Source: CAD feature listing. Evaluate the final solid. Frame: model axes, mm. A direction names the side the tool comes from. Give positions to 0.01 mm unless a question says otherwise; leave off trailing zeros. Order: outer loops, then holes, each group sorted by start corner. A loop starts at its lowest first (then second) coordinate and runs counter-clockwise, first axis right, second up. Notation, with made-up numbers: (54.25, -40) -> (69.25, -40) arc R20 cw to (69.25, -33) -> close; hole circle Ø10 at (84.5, -5.5). An arc over 180 degrees is marked (long way). Use CSV: the item, a comma, the result in double quotes.
```python
from build123d import *

# Parameters (mm, degrees)
SKETCH_1_R          = 2.1
EXTRUDE_1_DEPTH     = 5
SKETCH_2_R          = 3.75
EXTRUDE_2_DEPTH     = 4.2
SKETCH_3_R          = 4.35
EXTRUDE_3_DEPTH     = 1
SKETCH_9_R          = 2.5
CUT_EXTRUDE_1_DEPTH = 2.5


with BuildPart() as part:
    # 스케치1 → 보스-돌출1 (new body)
    with BuildSketch(Plane.XY):
        Circle(SKETCH_1_R)
    extrude(amount=EXTRUDE_1_DEPTH)

    # 스케치2 → 보스-돌출2 (add)
    with BuildSketch(Plane.XY.offset(5)):
        Circle(SKETCH_2_R)
    extrude(amount=EXTRUDE_2_DEPTH)

    # 스케치3 → 보스-돌출3 (add)
    with BuildSketch(Plane.XY.offset(9.2)):
        Circle(SKETCH_3_R)
    extrude(amount=EXTRUDE_3_DEPTH)

    # 스케치9 → 컷-돌출1 (cut)
    with BuildSketch(Plane.XY.offset(10.2)):
        Circle(SKETCH_9_R)
    extrude(amount=-CUT_EXTRUDE_1_DEPTH, mode=Mode.SUBTRACT)

    # 스케치13 → M2 남비 머리 나사용 카운터보어2 (revolve, cut)
    with BuildSketch(Plane(origin=(0, 0, 7.7), x_dir=(0, -1, 0), z_dir=(1, 0, 0))):
        Polygon((0, 0), (0, 8.781118805), (1.3, 8), (1.3, 1.6), (2.5, 1.6), (2.5, 0.025), (2.525, 0), align=None)
    revolve(axis=Axis((0, 0, 14.05), (0, 0, -1)), mode=Mode.SUBTRACT)


solid = part.part
```
1. Section query A-A on y = 0. Return loops of the section in (x, z) (3 decimals), plus the area to 3 significant figures.
Answer below:
outline,"(-4.35, 9.2) -> (-3.75, 9.2) -> (-3.75, 5) -> (-2.1, 5) -> (-2.1, 0) -> (-1.3, 0) -> (-1.3, 6.1) -> (-2.5, 6.1) -> (-2.5, 7.675) -> (-2.525, 7.7) -> (-2.5, 7.7) -> (-2.5, 10.2) -> (-4.35, 10.2) -> close; (1.3, 0) -> (2.1, 0) -> (2.1, 5) -> (3.75, 5) -> (3.75, 9.2) -> (4.35, 9.2) -> (4.35, 10.2) -> (2.5, 10.2) -> (2.5, 7.7) -> (2.525, 7.7) -> (2.5, 7.675) -> (2.5, 6.1) -> (1.3, 6.1) -> close"
area,"24.8 mm²"
2. Ray query, line 1 along Y through (x, z) = (0, 3.25); line 2 along Y through (x, z) = (0, 8.75); line 3 along Z through (x, y) = (-2.75, -0.75). Return the intervals inside material, ascending.
Answer below:
line 1,"y = -2.1 to -1.3, 1.3 to 2.1"
line 2,"y = -3.75 to -2.5, 2.5 to 3.75"
line 3,"z = 5 to 10.2"
3. Mould query, pull axis Y, two halves, no side actions, for faces 4 (the cylindrical face through (-0.943, -4.247, 9.693)), 5 (the flat face through (1, 4, 9.2)), 6 (the cylindrical face through (2.44, 0.54, 6.9)). Classes: released by +Y, released by -Y, zero draft, split by the parting line, or undercut.
Answer below:
face 4,"split by the parting line"
face 5,"zero draft"
face 6,"undercut"
4. Section query C-C on z = 8.25. Return loops of the section in (x, y).
Answer below:
outline,"circle Ø7.5 at (0, 0); hole circle Ø5 at (0, 0)"
5. Pin query (flat end, axial travel): P1, Ø5, axis at y = 0, z = 4.5, coming from the -X side; P2, Ø3.5, axis at x = 0, y = 0, coming from the +Z side; P3, Ø2, axis at x = 3.5, y = 1, coming from the -Z side; P4, Ø2.5, axis at x = -1, y = 0, coming from the -Z side. Return the tip coordinate at first contact, or that it passes through.
Answer below:
P1,"stops at x = -3.75"
P2,"stops at z = 6.1"
P3,"stops at z = 5"
P4,"stops at z = 0"
6. Section query D-D on z = 4. Return loops of the section in (x, y), plus the area to 3 significant figures.
Answer below:
outline,"circle Ø4.2 at (0, 0); hole circle Ø2.6 at (0, 0)"
area,"8.55 mm²"
7. Access query for faces 1 (the cylindrical face through (-0.54, -2.44, 8.97)), 2 (the flat face through (2, -2, 10.2)), 3 (the flat face through (2, -2, 5)). Directions: +Z, -Z, +X, -X, +Y, -Y. A direction counts if a zero-diameter tool reaches every point of the face in a straight line with its end or side. Return the directions, or none.
Answer below:
face 1,"+Z"
face 2,"+Z, +X, -X, +Y, -Y"
face 3,"-Z"
